For this review, take the finished solid that the model builds, in its own axes (mm). A direction names the side the tool comes from. Round coordinates to 2 decimals unless told otherwise and drop trailing zeros. Write each loop counter-clockwise with the first axis right and the second up, starting at its lowest first coordinate (ties: lowest second). Pieces come first, ordered by that corner, then holes. Notation, with made-up numbers: (48, -9) - (72, -9) arc R22 cw to (72, 3) - close; hole circle Ø2 at (-10.75, 14.25). An arc over 180 degrees is marked (long way). Answer in a Markdown table with one row per item. Add a question column.
from build123d import *

# Parameters (mm, degrees)
SKETCH1_R           = 3.302
BOSS_EXTRUDE1_DEPTH = 15.875
CUT_EXTRUDE1_DEPTH  = 12.7
SKETCH4_R           = 3.81
CUT_EXTRUDE2_DEPTH  = 13.97


with BuildPart() as part:
    # Sketch1 → Boss-Extrude1 (new body)
    with BuildSketch(Plane(origin=(0, 0, 0), x_dir=(1, 0, 0), z_dir=(0, 1, 0))):
        with BuildLine():
            Line((-98.396, 0), (98.396, 0))
            ThreePointArc((98.396, 0), (103.065733183, 1.934266817), (105, 6.604))
            Line((105, 6.604), (105, 153.396))
            ThreePointArc((105, 153.396), (103.065733183, 158.065733183), (98.396, 160))
            Line((98.396, 160), (-98.396, 160))
            ThreePointArc((-98.396, 160), (-103.065733183, 158.065733183), (-105, 153.396))
            Line((-105, 153.396), (-105, 6.604))
            ThreePointArc((-105, 6.604), (-103.065733183, 1.934266817), (-98.396, 0))
        make_face()
        with Locations(Location((-98.396, 6.604, 0), (0, 0, 270))):  # turned: the seam where the file's is
            Circle(SKETCH1_R, mode=Mode.SUBTRACT)
        with Locations(Location((98.396, 6.604, 0), (0, 0, 270))):  # turned: the seam where the file's is
            Circle(SKETCH1_R, mode=Mode.SUBTRACT)
        with Locations(Location((98.396, 153.396, 0), (0, 0, 270))):  # turned: the seam where the file's is
            Circle(SKETCH1_R, mode=Mode.SUBTRACT)
        with Locations(Location((-98.396, 153.396, 0), (0, 0, 270))):  # turned: the seam where the file's is
            Circle(SKETCH1_R, mode=Mode.SUBTRACT)
    extrude(amount=BOSS_EXTRUDE1_DEPTH)

    # Sketch3 → Cut-Extrude1 (cut)
    with BuildSketch(Plane(origin=(0, 15.875, 0), x_dir=(1, 0, 0), z_dir=(0, 1, 0))):
        with BuildLine():
            Line((63.598, 80.01), (63.598, 81.28))
            ThreePointArc((63.598, 81.28), (52.289978608, 108.579978608), (24.99, 119.888))
            Line((24.99, 119.888), (-61.185, 119.888))
            ThreePointArc((-61.185, 119.888), (-63.598, 117.475), (-61.185, 115.062))
            Line((-61.185, 115.062), (24.99, 115.062))
            ThreePointArc((24.99, 115.062), (59.407, 80.645), (24.99, 46.228))
            Line((24.99, 46.228), (-61.185, 46.228))
            ThreePointArc((-61.185, 46.228), (-63.598, 43.815), (-61.185, 41.402))
            Line((-61.185, 41.402), (-12.729, 41.402))
            ThreePointArc((-12.729, 41.402), (3.273, 25.4), (-12.729, 9.398))
            Line((-12.729, 9.398), (-61.185, 9.398))
            ThreePointArc((-61.185, 9.398), (-95.602, 43.815), (-61.185, 78.232))
            Line((-61.185, 78.232), (24.99, 78.232))
            ThreePointArc((24.99, 78.232), (27.403, 80.645), (24.99, 83.058))
            Line((24.99, 83.058), (-61.185, 83.058))
            ThreePointArc((-61.185, 83.058), (-95.602, 117.475), (-61.185, 151.892))
            Line((-61.185, 151.892), (24.99, 151.892))
            ThreePointArc((24.99, 151.892), (74.920224033, 131.210224033), (95.602, 81.28))
            Line((95.602, 81.28), (95.602, 80.01))
            ThreePointArc((95.602, 80.01), (74.920224033, 30.079775967), (24.99, 9.398))
            Line((24.99, 9.398), (22.831, 9.398))
            ThreePointArc((22.831, 9.398), (6.829, 25.4), (22.831, 41.402))
            Line((22.831, 41.402), (24.99, 41.402))
            ThreePointArc((24.99, 41.402), (52.289978608, 52.710021392), (63.598, 80.01))
        make_face()
    extrude(amount=-CUT_EXTRUDE1_DEPTH, mode=Mode.SUBTRACT)

    # Sketch4 → Cut-Extrude2 (cut)
    with BuildSketch(Plane.XY):
        with Locations((-13.941, 7.9375)):
            Circle(SKETCH4_R)
        with Locations((24.159, 7.9375)):
            Circle(SKETCH4_R)
    extrude(amount=-CUT_EXTRUDE2_DEPTH, mode=Mode.SUBTRACT)


solid = part.part
Q1. Tool access review of faces 5 (the face through (-17, 10, -83.058)), 6 (the face through (-1, 8, 0)): name each direction out of +Z, -Z, +X, -X, +Y, -Y from which nothing blocks a thin tool from reaching the whole face with its end or side.
Q2. Draft analysis for pull direction X (two halves, no side actions). For faces 1 (the face through (74.368, 9.614, -131.756)), 2 (the face through (1, 8, -160)), 3 (the face through (6.833, 9.614, -25.048)), 4 (the face through (-103.12, 7.83, -1.99)), state which applies: released by +X, released by -X, zero draft, split by the parting line, or undercut.
Q3. Add section C-C on z = -25.4. State the section outline as (x, y) points (3 decimals), then the cut area to 3 significant figures.
Q4. Add section A-A on x = -44. State the section outline as (y, z) points (3 decimals), then the cut area to 3 significant figures.
Q5. Add section B-B on z = -86. State the section outline as (x, y) points (3 decimals), then the cut area to 3 significant figures.
Q6. Add section D-D on z = -140. State the section outline as (x, y) points (3 decimals).
Q7. To check wall thickness, follow probe 1 along Z at (x, y) = (-14, 7.5); probe 2 along X at (y, z) = (14.75, -81); probe 3 along Z at (x, y) = (-90.5, 12.75). State the ranges of each line that lie inside material, in increasing order.
Q8. Insertion check: pin 1 Ø4 at (x, z) = (98.396, -153.396) entering from +Y; pin 2 Ø4.5 at (x, y) = (24.16, 7.94) entering from +Z; pin 3 Ø3 at (x, z) = (12, -130.5) entering from +Y (3 decimals). Each pin has a flat end and moves straight along its axis. Give the tip position at first contact, or say it passes through.
Answer sheet:
| question | item | result |
|---|---|---|
| 1 | face 5 | +Y |
| 1 | face 6 | +Z, +X, -X, +Y, -Y |
| 2 | face 1 | undercut |
| 2 | face 2 | zero draft |
| 2 | face 3 | undercut |
| 2 | face 4 | released by -X |
| 3 | outline | (-105, 0) - (105, 0) - (105, 15.875) - (69.754, 15.875) - (69.754, 3.175) - (6.829, 3.175) - (6.829, 15.875) - (3.273, 15.875) - (3.273, 3.175) - (-90.261, 3.175) - (-90.261, 15.875) - (-105, 15.875) - close |
| 3 | area | 1,350 mm² |
| 4 | outline | (0, -160) - (15.875, -160) - (15.875, -151.892) - (3.175, -151.892) - (3.175, -119.888) - (15.875, -119.888) - (15.875, -115.062) - (3.175, -115.062) - (3.175, -83.058) - (15.875, -83.058) - (15.875, -78.232) - (3.175, -78.232) - (3.175, -46.228) - (15.875, -46.228) - (15.875, -41.402) - (3.175, -41.402) - (3.175, -9.398) - (15.875, -9.398) - (15.875, 0) - (0, 0) - close |
| 4 | area | 914 mm² |
| 5 | outline | (-105, 0) - (105, 0) - (105, 15.875) - (95.444, 15.875) - (95.444, 3.175) - (63.308, 3.175) - (63.308, 15.875) - (58.988, 15.875) - (58.988, 3.175) - (-75.108, 3.175) - (-75.108, 15.875) - (-105, 15.875) - close |
| 5 | area | 1,220 mm² |
| 6 | outline | (-105, 0) - (105, 0) - (105, 15.875) - (64.208, 15.875) - (64.208, 3.175) - (-87.207, 3.175) - (-87.207, 15.875) - (-105, 15.875) - close |
| 7 | probe 1 | z = -160 to -151.89, -119.89 to -115.06, -83.06 to -78.23, -46.23 to -41.4 |
| 7 | probe 2 | x = -105 to 27.38, 59.41 to 63.6, 95.6 to 105 |
| 7 | probe 3 | z = -160 to -135.51, -99.44 to -61.85, -25.78 to 0 |
| 8 | pin 1 | passes through |
| 8 | pin 2 | stops at z = -41.38 |
| 8 | pin 3 | stops at y = 3.175 |
